Geometry: see drawing. Coordinates: mm, zero at the bounding-box minimum. Round coordinates to 2 decimals unless told otherwise and drop trailing zeros. Write each loop counter-clockwise with the first axis right and the second up, starting at its lowest first coordinate (ties: lowest second). Pieces come first, ordered by that corner, then holes.
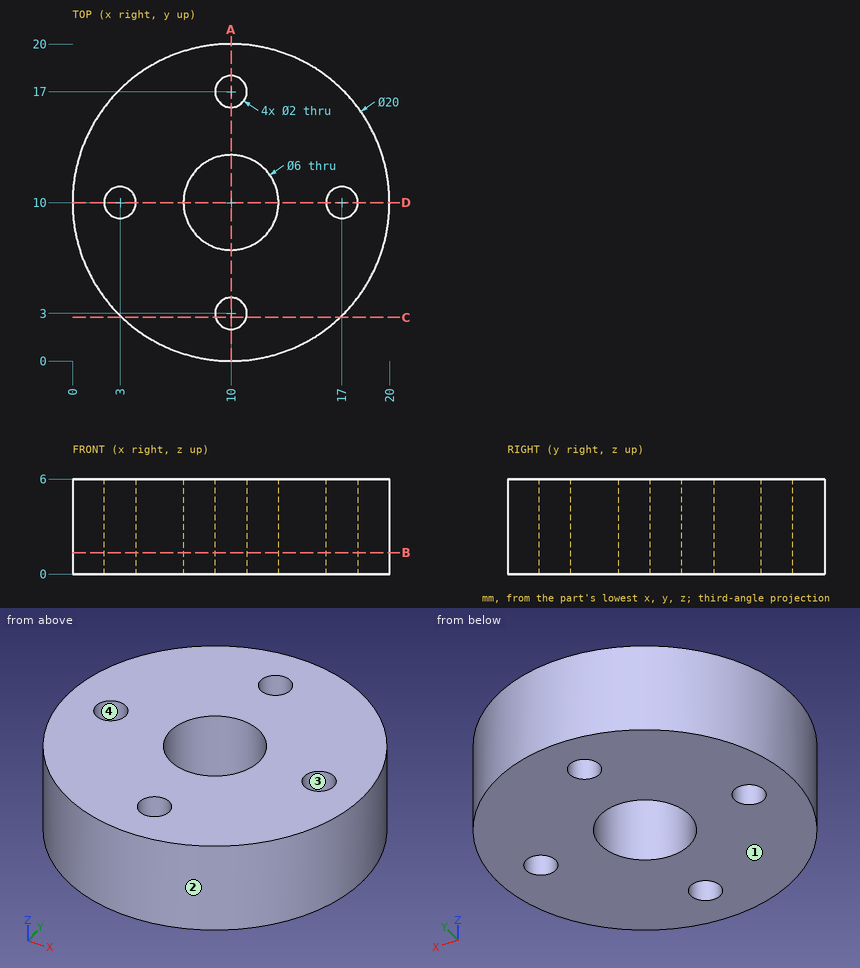
Q1. Section query B-B, the plane z = 1.35. Output: boundary loops of the cut face in (x, y), and give its area (3 significant figures).
Q2. Line query: line 1 (Y direction, x = 10, z = 1.9); line 2 (X direction, y = 2.5, z = 4.75); line 3 (Y direction, x = 17, z = 3.2). Output: solid intervals per line, ascending.
Q3. Section query A-A, the plane x = 10. Output: boundary loops of the cut face in (y, z), and give its area (3 significant figures).
Q4. Section query C-C, the plane y = 2.75. Output: boundary loops of the cut face in (x, z), and give its area (3 significant figures).
Q5. Mould query, pull axis X, two halves, no side actions, for the marked faces 1, 2, 3 and 4. Classes: pulls with the +X half, pulls with the -X half, needs draft (parallel to the pull), parting line crosses it, or undercut.
Q6. Pin query (flat end, axial travel): P1, Ø2.5, axis at x = 10, y = 17, coming from the -Z side; P2, Ø1.5, axis at y = 17.5, z = 2, coming from the +X side; P3, Ø3, axis at x = 17, z = 4.5, coming from the -Y side. Return the tip coordinate at first contact, or that it passes through.
Filled in:
1. outline: circle Ø20 at (10, 10); hole circle Ø2 at (3, 10); hole circle Ø6 at (10, 10); hole circle Ø2 at (10, 3); hole circle Ø2 at (10, 17); hole circle Ø2 at (17, 10)
1. area: 273 mm2
2. line 1: y = 0 to 2, 4 to 7, 13 to 16, 18 to 20
2. line 2: x = 3.39 to 9.13, 10.87 to 16.61
2. line 3: y = 2.86 to 9, 11 to 17.14
3. outline: (0, 0) - (2, 0) - (2, 6) - (0, 6) - close; (4, 0) - (7, 0) - (7, 6) - (4, 6) - close; (13, 0) - (16, 0) - (16, 6) - (13, 6) - close; (18, 0) - (20, 0) - (20, 6) - (18, 6) - close
3. area: 60.0 mm2
4. outline: (3.11, 0) - (9.03, 0) - (9.03, 6) - (3.11, 6) - close; (10.97, 0) - (16.89, 0) - (16.89, 6) - (10.97, 6) - close
4. area: 71.0 mm2
5. face 1: needs draft
5. face 2: parting line crosses it
5. face 3: undercut
5. face 4: undercut
6. P1: stops at z = 0
6. P2: stops at x = 17.38
6. P3: stops at y = 1.65
